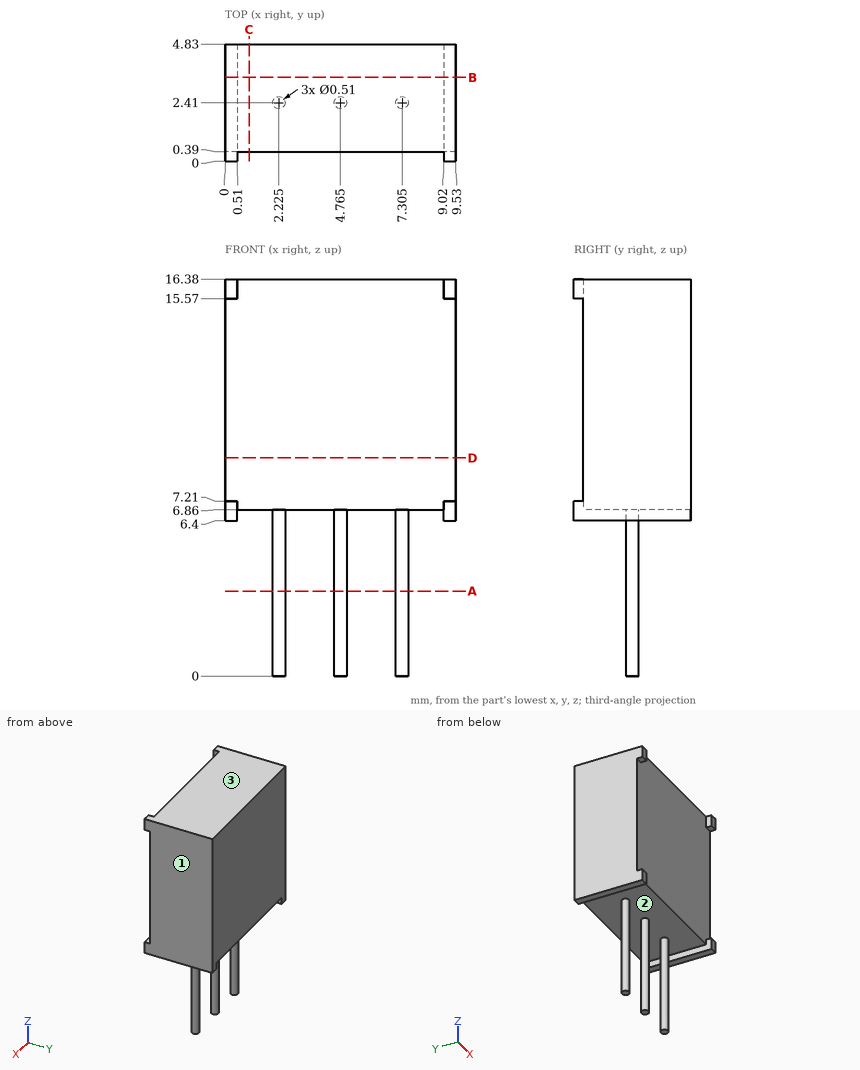
Could you check a few things on this drawing? It's one solid part, dimensions in mm from its lowest x, y, z. Round coordinates to 2 decimals unless told otherwise and drop trailing zeros. Write each loop counter-clockwise with the first axis right and the second up, starting at its lowest first coordinate (ties: lowest second). Pieces come first, ordered by that corner, then holes. Notation, with made-up numbers: M -24.75,42.25 L 31.25,42.25 A33 cw 31.25,73.25 Z; hole C 61.5,29.25 d3. An arc over 180 degrees is marked long. Answer as CSV lines item,"result". Start each with the question number.
1. Suppose I cut it at C-C on x = 1. Write out the boundary of the cut face in (y, z).
2. I need wall thicknesses on probe 1 along X at (y, z) = (2.3, 5.75); probe 2 along X at (y, z) = (4.45, 6.5); probe 3 along Y at (x, z) = (4.25, 8.5). Which ranges of each line are inside material? Lowest first, please.
3. Suppose I cut it at A-A on z = 3.5. Write out the boundary of the cut face in (x, y) (3 decimals), then the cut area to 3 significant figures.
4. Thinking about a two-plate mould opening in X: for the marked faces 1, 2 and 3, which applies, released by +X, released by -X, zero draft, split by the parting line, or undercut?
5. Suppose I cut it at B-B on y = 3.45. Write out the boundary of the cut face in (x, z).
6. Suppose I cut it at D-D on z = 9. Write out the boundary of the cut face in (x, y), then the cut area to 3 significant figures.
7. I'm going to push flat-ended pins straight in: pin 1 Ø2 at (y, z) = (0.5, 3.5) entering from -X; pin 2 Ø1 at (x, y) = (3, 3) entering from -Z; pin 3 Ø1.5 at (x, z) = (6.5, 4.5) entering from +Y. Where does each tip first touch, or does it pass through?
Check result:
1,outline,"M 0.39,6.86 L 4.83,6.86 L 4.83,16.38 L 0.39,16.38 Z"
2,probe 1,"x = 1.99 to 2.46, 4.53 to 5, 7.07 to 7.54"
2,probe 2,"x = 0 to 0.51, 9.02 to 9.53"
2,probe 3,"y = 0.39 to 4.83"
3,outline,"C 2.225,2.41 d0.51; C 4.765,2.41 d0.51; C 7.305,2.41 d0.51"
3,area,"0.613 mm2"
4,face 1,"released by +X"
4,face 2,"undercut"
4,face 3,"zero draft"
5,outline,"M 0,6.4 L 0.51,6.4 L 0.51,6.86 L 9.02,6.86 L 9.02,6.4 L 9.53,6.4 L 9.53,16.38 L 0,16.38 Z"
6,outline,"M 0,0.39 L 9.53,0.39 L 9.53,4.83 L 0,4.83 Z"
6,area,"42.3 mm2"
7,pin 1,"passes through"
7,pin 2,"stops at z = 6.86"
7,pin 3,"stops at y = 2.66"
